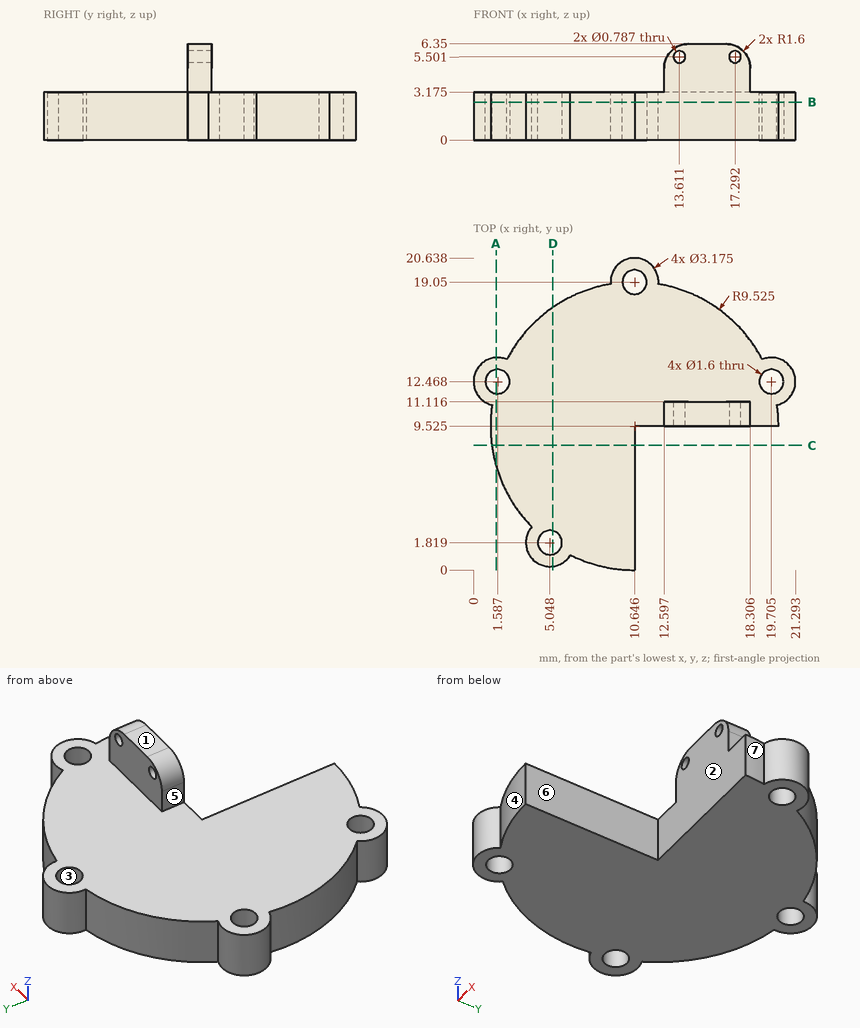
Answer from the drawing. Dimensions are ordinates in mm from the lowest x, y and z of the part. A direction names the side the tool comes from. Round coordinates to 2 decimals unless told otherwise and drop trailing zeros. Loops run counter-clockwise (first coordinate to the right, second up) from the corner with the lowest first, then second, coordinate; pieces in that order, holes last.
(1) Find the intervals of material crossed by L1, parallel to X at y = 12.25, z = 1 (1 decimal); L2, parallel to Z at x = 8.5, y = 4.25 (1 decimal); L3, parallel to Y at x = 5.25, z = 1.5 (1 decimal), in increasing order.
Computed values:
L1: x = 0 to 0.8, 2.4 to 18.9, 20.5 to 21.3
L2: z = 0 to 3.2
L3: y = 0.2 to 1, 2.6 to 17.4
(2) The part is cut by section D-D, the plane x = 5.25. Give the vertices of the cut face in (y, z) (1 decimal).
Computed values:
outline: (0.2, 0) - (1, 0) - (1, 3.2) - (0.2, 3.2) - close; (2.6, 0) - (17.4, 0) - (17.4, 3.2) - (2.6, 3.2) - close
(3) For the marked faces 4, 5, 6 and 7, determine the directions among +Z, -Z, +X, -X, +Y, -Y from which every point of the face is accessible in a straight line to the end or side of a thin tool.
Computed values:
face 4: +Z, -Z, -Y
face 5: +Z, -X, +Y, -Y
face 6: +Z, -Z, +X, -Y
face 7: +Z, -Z, +X
(4) The part is cut by section A-A, the plane x = 1.5. Give the vertices of the cut face in (y, z) (1 decimal).
Computed values:
outline: (6.9, 0) - (11.7, 0) - (11.7, 3.2) - (6.9, 3.2) - close; (13.3, 0) - (14.1, 0) - (14.1, 3.2) - (13.3, 3.2) - close
(5) The part is cut by section B-B, the plane z = 2.5. Give the number of separate pieces and of enclosed holes in the cut face, and give its area (3 significant figures).
Computed values:
separate pieces: 1
enclosed holes: 4
area: 222 mm2
(6) Each of these flat-tipped pins is pushed along its axis until it touches: P1, Ø2, axis at x = 17, y = 17.5, coming from the +Z side (1 decimal); P2, Ø0.5, axis at y = 10, z = 3.5, coming from the +X side; P3, Ø3.5, axis at y = 7, z = 2, coming from the +X side; P4, Ø1, axis at x = 10.65, y = 19.05, coming from the -Z side. Where does it stop, or does it pass through?
Computed values:
P1: stops at z = 3.2
P2: stops at x = 18.31
P3: stops at x = 10.65
P4: passes through
(7) The mould has two halves that part along Y. Classify the marked faces 1, 2 and 3: pulls with the +Y half, pulls with the -Y half, needs draft (parallel to the pull), parting line crosses it, or undercut.
Computed values:
face 1: needs draft
face 2: pulls with the -Y half
face 3: undercut
(8) The part is cut by section C-C, the plane y = 8.25. Give the vertices of the cut face in (x, z) (1 decimal).
Computed values:
outline: (1.2, 0) - (10.6, 0) - (10.6, 3.2) - (1.2, 3.2) - close
